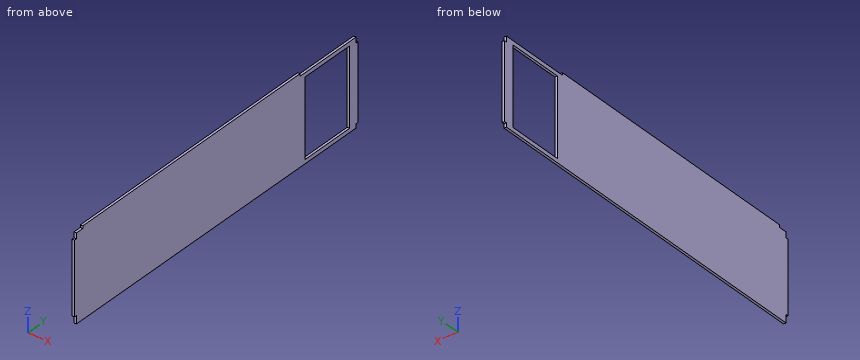
Autodesk Inventor part; units mm, degrees
ref_plane "YZ Plane" through (0, 0, 0) normal (1, 0, 0) x (0, 1, 0)
ref_plane "XZ Plane" through (0, 0, 0) normal (0, 1, 0) x (-1, 0, 0)
ref_plane "XY Plane" through (0, 0, 0) normal (0, 0, 1) x (1, 0, 0)
sketch "Sketch1" plane through (0, 0, 0) normal (1, 0, 0) x (0, 1, 0)
  line L0 (0, 0) -> (442, 0)
  line L1 (442, 0) -> (442, -110)
  line L2 (442, -110) -> (0, -110)
  line L3 (0, -110) -> (0, 0)
  line L4 (3, 0) -> (3, -10)
  line L5 (3, -10) -> (0, -10)
  line L6 (3, -110) -> (3, -100)
  line L7 (3, -100) -> (0, -100)
  line L8 (13, 0) -> (13, -3)
  line L9 (13, -3) -> (3, -3)
  line L10 (442, -3) -> (354, -3)
  line L11 (354, -3) -> (354, 0)
  dimension "d0" = 442
  dimension "d1" = 110
  dimension "d2" = 3
  dimension "d3" = 10
  dimension "d4" = 10
  dimension "d5" = 10
  dimension "d6" = 3
  dimension "d7" = 88
  dimension "d8" = 3
extrude "Extrusion1" add sketch "Sketch1" along normal blind 3 contours L5 L4 L9 L8 L0 L11 L10 L1 L2 L6 L7 L3
sketch "Sketch2" plane through (0, 442, -3) normal (0, 1, 0) x (1, 0, 0)
  line L0 (0, 7) -> (0, 97)
  line L1 (0, 7) -> (3, 7)
  line L2 (3, 7) -> (3, 97)
  line L3 (0, 7) -> (0, 102)
  line L4 (0, 97) -> (0, 107)
  line L5 (3, 97) -> (3, 107)
  line L6 (3, 102) -> (0, 102)
  line L7 (3, 102) -> (3, 7)
  line L8 (0, 7) -> (3, 7)
  line L9 (0, 107) -> (3, 107)
  line L10 (0, 0) -> (3, 0)
  point P0 (0, -3)
  point P1 (0, 97)
  dimension "d12" = 5
  dimension "d15" = 7
extrude "Extrusion2" add sketch "Sketch2" along normal blind 3 contours L0 L3 L6 L5 L2 L1
sketch "Sketch3" plane through (3, 0, 0) normal (1, 0, 0) x (0, 0, -1)
  line L0 (8, 432) -> (8, 362)
  line L1 (8, 362) -> (105, 362)
  line L2 (105, 362) -> (105, 432)
  line L3 (105, 432) -> (8, 432)
  line L4 (3, 442) -> (3, 354)
  line L5 (110, 3) -> (110, 442)
  line L6 (10, 445) -> (105, 445)
  point P0 (0, 0)
  dimension "d16" = 5
  dimension "d17" = 5
  dimension "d18" = 70
  dimension "d19" = 13
extrude "Extrusion3" cut sketch "Sketch3" against normal blind 3
properties part number "Lift cover of lifting" material "PMMA Plastic"
Check sheet for the modelled part. Datum: model origin and axes. Units: mm. Round coordinates to 2 decimals unless told otherwise and drop trailing zeros. Order: outer loops, then holes, each group sorted by start corner. A loop starts at its lowest first (then second) coordinate and runs counter-clockwise, first axis right, second up.
1) Scan lines: line 1 (Y direction, x = 1.55, z = -18); line 2 (Z direction, x = 1.2, y = 387.5); line 3 (Y direction, x = 2.2, z = -104.5). Record each from-to range of solid material in increasing order.
2) Section check B-B (x = 2.25). Record the boundary of the cut face in (y, z).
3) Go/stop test with flat-tipped pins: pin 1 Ø0.9 at (x, y) = (2, 443) entering from -Z; pin 2 Ø1.5 at (x, y) = (1, 393.5) entering from +Z; pin 3 Ø1.5 at (x, y) = (1.5, 2) entering from -Z. Record where each tip stops, or that it passes through.
4) Section check A-A (z = -94.5). Record the boundary of the cut face in (x, y), and give its area (4 significant figures).
Result:
1. line 1: y = 0 to 362, 432 to 445
1. line 2: z = -110 to -105, -8 to -3
1. line 3: y = 3 to 362, 432 to 445
2. outline: (0, -100) - (3, -100) - (3, -110) - (442, -110) - (442, -105) - (445, -105) - (445, -10) - (442, -10) - (442, -3) - (354, -3) - (354, 0) - (13, 0) - (13, -3) - (3, -3) - (3, -10) - (0, -10) - close; hole (362, -105) - (432, -105) - (432, -8) - (362, -8) - close
3. pin 1: stops at z = -105
3. pin 2: stops at z = -3
3. pin 3: stops at z = -100
4. outline: (0, 0) - (3, 0) - (3, 362) - (0, 362) - close; (0, 432) - (3, 432) - (3, 445) - (0, 445) - close
4. area: 1,125 mm2
